from build123d import *

# Parameters (mm, degrees)
SKETCH1_R                 = 5.6
BOSS_EXTRUDE1_DEPTH       = 3
CUT_EXTRUDE1_START        = -3
CUT_EXTRUDE1_DEPTH        = 3
CIRPATTERN1_COUNT         = 12
CIRPATTERN1_START         = -3
CIRPATTERN1_COPY_1_DEPTH  = 3
CIRPATTERN1_COPY_2_DEPTH  = 3
CIRPATTERN1_COPY_3_DEPTH  = 3
CIRPATTERN1_COPY_4_DEPTH  = 3
CIRPATTERN1_COPY_5_DEPTH  = 3
CIRPATTERN1_COPY_6_DEPTH  = 3
CIRPATTERN1_COPY_7_DEPTH  = 3
CIRPATTERN1_COPY_8_DEPTH  = 3
CIRPATTERN1_COPY_9_DEPTH  = 3
CIRPATTERN1_COPY_10_DEPTH = 3
CIRPATTERN1_COPY_11_DEPTH = 3


with BuildPart() as part:
    # Sketch1 → Boss-Extrude1 (new body)
    with BuildSketch(Plane(origin=(0, 0, 0), x_dir=(1, 0, 0), z_dir=(0, 1, 0))):
        with Locations(Location((0, 0, 0), (0, 0, 270))):
            Circle(SKETCH1_R)
    extrude(amount=BOSS_EXTRUDE1_DEPTH)

    # Sketch2 → Cut-Extrude1 (cut)
    with BuildSketch(Plane(origin=(0, 3, 0), x_dir=(1, 0, 0), z_dir=(0, 1, 0)).offset(CUT_EXTRUDE1_START)):
        with BuildLine():
            Line((0.510357412, 3.876549408), (0.730946676, 5.552091224))
            ThreePointArc((0.730946676, 5.552091224), (0.075009446, 5.599497619), (-0.581962275, 5.569678618))
            ThreePointArc((-0.581962275, 5.569678618), (-0.013232679, 4.835071359), (0.066186197, 3.909439779))
            ThreePointArc((0.066186197, 3.909439779), (0.288740502, 3.899324162), (0.510357412, 3.876549408))
        make_face()
    cut_extrude1 = extrude(amount=CUT_EXTRUDE1_DEPTH, mode=Mode.SUBTRACT)

    # Mirror1: Cut-Extrude1 across plane
    add(cut_extrude1.mirror(Plane(origin=(0, 0, 0), x_dir=(-0.13052619222004483, 0, 0.9914448613738113), z_dir=(-0.9914448613738114, 0, -0.13052619222004483))), mode=Mode.SUBTRACT)

    # CirPattern1: Cut-Extrude1 ×12 about axis
    cirpattern1_axis = Axis((0, 0, 0), (0, 1, 0))
    for i in range(1, CIRPATTERN1_COUNT):
        add(cut_extrude1.rotate(cirpattern1_axis, i * 360 / CIRPATTERN1_COUNT), mode=Mode.SUBTRACT)

    # CirPattern1 copy 1 sketch → CirPattern1 copy 1 (cut)
    with BuildSketch(Plane(origin=(0, 3, 0), x_dir=(-0.9659258262890651, 0, 0.25881904510253406), z_dir=(0, 1, 0)).offset(CIRPATTERN1_START)):
        with BuildLine():
            Line((0.510357412, -3.876549408), (0.730946676, -5.552091224))
            ThreePointArc((0.730946676, -5.552091224), (0.075009446, -5.599497619), (-0.581962275, -5.569678618))
            ThreePointArc((-0.581962275, -5.569678618), (-0.013232679, -4.835071359), (0.066186197, -3.909439779))
            ThreePointArc((0.066186197, -3.909439779), (0.288740502, -3.899324162), (0.510357412, -3.876549408))
        make_face()
    extrude(amount=CIRPATTERN1_COPY_1_DEPTH, mode=Mode.SUBTRACT)

    # CirPattern1 copy 2 sketch → CirPattern1 copy 2 (cut)
    with BuildSketch(Plane(origin=(0, 3, 0), x_dir=(-0.7071067811865381, 0, 0.7071067811865575), z_dir=(0, 1, 0)).offset(CIRPATTERN1_START)):
        with BuildLine():
            Line((0.510357412, -3.876549408), (0.730946676, -5.552091224))
            ThreePointArc((0.730946676, -5.552091224), (0.075009446, -5.599497619), (-0.581962275, -5.569678618))
            ThreePointArc((-0.581962275, -5.569678618), (-0.013232679, -4.835071359), (0.066186197, -3.909439779))
            ThreePointArc((0.066186197, -3.909439779), (0.288740502, -3.899324162), (0.510357412, -3.876549408))
        make_face()
    extrude(amount=CIRPATTERN1_COPY_2_DEPTH, mode=Mode.SUBTRACT)

    # CirPattern1 copy 3 sketch → CirPattern1 copy 3 (cut)
    with BuildSketch(Plane(origin=(0, 3, 0), x_dir=(-0.25881904510250764, 0, 0.9659258262890722), z_dir=(0, 1, 0)).offset(CIRPATTERN1_START)):
        with BuildLine():
            Line((0.510357412, -3.876549408), (0.730946676, -5.552091224))
            ThreePointArc((0.730946676, -5.552091224), (0.075009446, -5.599497619), (-0.581962275, -5.569678618))
            ThreePointArc((-0.581962275, -5.569678618), (-0.013232679, -4.835071359), (0.066186197, -3.909439779))
            ThreePointArc((0.066186197, -3.909439779), (0.288740502, -3.899324162), (0.510357412, -3.876549408))
        make_face()
    extrude(amount=CIRPATTERN1_COPY_3_DEPTH, mode=Mode.SUBTRACT)

    # CirPattern1 copy 4 sketch → CirPattern1 copy 4 (cut)
    with BuildSketch(Plane(origin=(0, 3, 0), x_dir=(0.2588190451025339, 0, 0.9659258262890651), z_dir=(0, 1, 0)).offset(CIRPATTERN1_START)):
        with BuildLine():
            Line((0.510357412, -3.876549408), (0.730946676, -5.552091224))
            ThreePointArc((0.730946676, -5.552091224), (0.075009446, -5.599497619), (-0.581962275, -5.569678618))
            ThreePointArc((-0.581962275, -5.569678618), (-0.013232679, -4.835071359), (0.066186197, -3.909439779))
            ThreePointArc((0.066186197, -3.909439779), (0.288740502, -3.899324162), (0.510357412, -3.876549408))
        make_face()
    extrude(amount=CIRPATTERN1_COPY_4_DEPTH, mode=Mode.SUBTRACT)

    # CirPattern1 copy 5 sketch → CirPattern1 copy 5 (cut)
    with BuildSketch(Plane(origin=(0, 3, 0), x_dir=(0.7071067811865577, 0, 0.707106781186538), z_dir=(0, 1, 0)).offset(CIRPATTERN1_START)):
        with BuildLine():
            Line((0.510357412, -3.876549408), (0.730946676, -5.552091224))
            ThreePointArc((0.730946676, -5.552091224), (0.075009446, -5.599497619), (-0.581962275, -5.569678618))
            ThreePointArc((-0.581962275, -5.569678618), (-0.013232679, -4.835071359), (0.066186197, -3.909439779))
            ThreePointArc((0.066186197, -3.909439779), (0.288740502, -3.899324162), (0.510357412, -3.876549408))
        make_face()
    extrude(amount=CIRPATTERN1_COPY_5_DEPTH, mode=Mode.SUBTRACT)

    # CirPattern1 copy 6 sketch → CirPattern1 copy 6 (cut)
    with BuildSketch(Plane(origin=(0, 3, 0), x_dir=(0.9659258262890722, 0, 0.2588190451025077), z_dir=(0, 1, 0)).offset(CIRPATTERN1_START)):
        with BuildLine():
            Line((0.510357412, -3.876549408), (0.730946676, -5.552091224))
            ThreePointArc((0.730946676, -5.552091224), (0.075009446, -5.599497619), (-0.581962275, -5.569678618))
            ThreePointArc((-0.581962275, -5.569678618), (-0.013232679, -4.835071359), (0.066186197, -3.909439779))
            ThreePointArc((0.066186197, -3.909439779), (0.288740502, -3.899324162), (0.510357412, -3.876549408))
        make_face()
    extrude(amount=CIRPATTERN1_COPY_6_DEPTH, mode=Mode.SUBTRACT)

    # CirPattern1 copy 7 sketch → CirPattern1 copy 7 (cut)
    with BuildSketch(Plane(origin=(0, 3, 0), x_dir=(0.9659258262890651, 0, -0.2588190451025343), z_dir=(0, 1, 0)).offset(CIRPATTERN1_START)):
        with BuildLine():
            Line((0.510357412, -3.876549408), (0.730946676, -5.552091224))
            ThreePointArc((0.730946676, -5.552091224), (0.075009446, -5.599497619), (-0.581962275, -5.569678618))
            ThreePointArc((-0.581962275, -5.569678618), (-0.013232679, -4.835071359), (0.066186197, -3.909439779))
            ThreePointArc((0.066186197, -3.909439779), (0.288740502, -3.899324162), (0.510357412, -3.876549408))
        make_face()
    extrude(amount=CIRPATTERN1_COPY_7_DEPTH, mode=Mode.SUBTRACT)

    # CirPattern1 copy 8 sketch → CirPattern1 copy 8 (cut)
    with BuildSketch(Plane(origin=(0, 3, 0), x_dir=(0.7071067811865385, 0, -0.7071067811865571), z_dir=(0, 1, 0)).offset(CIRPATTERN1_START)):
        with BuildLine():
            Line((0.510357412, -3.876549408), (0.730946676, -5.552091224))
            ThreePointArc((0.730946676, -5.552091224), (0.075009446, -5.599497619), (-0.581962275, -5.569678618))
            ThreePointArc((-0.581962275, -5.569678618), (-0.013232679, -4.835071359), (0.066186197, -3.909439779))
            ThreePointArc((0.066186197, -3.909439779), (0.288740502, -3.899324162), (0.510357412, -3.876549408))
        make_face()
    extrude(amount=CIRPATTERN1_COPY_8_DEPTH, mode=Mode.SUBTRACT)

    # CirPattern1 copy 9 sketch → CirPattern1 copy 9 (cut)
    with BuildSketch(Plane(origin=(0, 3, 0), x_dir=(0.25881904510250775, 0, -0.9659258262890722), z_dir=(0, 1, 0)).offset(CIRPATTERN1_START)):
        with BuildLine():
            Line((0.510357412, -3.876549408), (0.730946676, -5.552091224))
            ThreePointArc((0.730946676, -5.552091224), (0.075009446, -5.599497619), (-0.581962275, -5.569678618))
            ThreePointArc((-0.581962275, -5.569678618), (-0.013232679, -4.835071359), (0.066186197, -3.909439779))
            ThreePointArc((0.066186197, -3.909439779), (0.288740502, -3.899324162), (0.510357412, -3.876549408))
        make_face()
    extrude(amount=CIRPATTERN1_COPY_9_DEPTH, mode=Mode.SUBTRACT)

    # CirPattern1 copy 10 sketch → CirPattern1 copy 10 (cut)
    with BuildSketch(Plane(origin=(0, 3, 0), x_dir=(-0.2588190451025343, 0, -0.9659258262890651), z_dir=(0, 1, 0)).offset(CIRPATTERN1_START)):
        with BuildLine():
            Line((0.510357412, -3.876549408), (0.730946676, -5.552091224))
            ThreePointArc((0.730946676, -5.552091224), (0.075009446, -5.599497619), (-0.581962275, -5.569678618))
            ThreePointArc((-0.581962275, -5.569678618), (-0.013232679, -4.835071359), (0.066186197, -3.909439779))
            ThreePointArc((0.066186197, -3.909439779), (0.288740502, -3.899324162), (0.510357412, -3.876549408))
        make_face()
    extrude(amount=CIRPATTERN1_COPY_10_DEPTH, mode=Mode.SUBTRACT)

    # CirPattern1 copy 11 sketch → CirPattern1 copy 11 (cut)
    with BuildSketch(Plane(origin=(0, 3, 0), x_dir=(-0.7071067811865571, 0, -0.7071067811865385), z_dir=(0, 1, 0)).offset(CIRPATTERN1_START)):
        with BuildLine():
            Line((0.510357412, -3.876549408), (0.730946676, -5.552091224))
            ThreePointArc((0.730946676, -5.552091224), (0.075009446, -5.599497619), (-0.581962275, -5.569678618))
            ThreePointArc((-0.581962275, -5.569678618), (-0.013232679, -4.835071359), (0.066186197, -3.909439779))
            ThreePointArc((0.066186197, -3.909439779), (0.288740502, -3.899324162), (0.510357412, -3.876549408))
        make_face()
    extrude(amount=CIRPATTERN1_COPY_11_DEPTH, mode=Mode.SUBTRACT)


solid = part.part
Design review of the part built by this model. Coordinates are the model's own, in mm. A direction names the side the tool comes from. Round coordinates to 2 decimals unless told otherwise and drop trailing zeros. Order: outer loops, then holes, each group sorted by start corner. A loop starts at its lowest first (then second) coordinate and runs counter-clockwise, first axis right, second up. Notation, with made-up numbers: M 11,23 L 27,23 A23 cw 27,47 Z; hole C 23,29 d3. An arc over 180 degrees is marked long. Answer as CSV lines item,"result". Start each with the question number.
1) Wall thickness on line 1 along X through (y, z) = (1.05, 4.25); line 2 along Z through (x, y) = (3, 1.25); line 3 along Z through (x, y) = (-3, 0.4): over which ranges is each line inside the solid? List them lowest first. Write a range as [from, to].
2) The part is to be moulded in two halves that separate along X. For faces 3 (the face through (0, 3, 0)), 4 (the face through (-1.272, 1.479, 4.677)), say which applies: +X half, -X half, draft (parallel to the pull), parting line (faces both ways), or undercut.
3) Add section B-B (x = 1.75). Give the boundary of the cut face in (y, z), then the cut area to 3 significant figures.
4) Tool access review of faces 1 (the face through (4.677, 1.479, 1.272)), 2 (the face through (0, 0, 0)): name each direction out of +Z, -Z, +X, -X, +Y, -Y from which nothing blocks a thin tool from reaching the whole face with its end or side.
5) For pin 1 Ø1 at (x, y) = (-4, 2.5) entering from +Z, flat-tipped, find the tip position at first contact; note if it passes through.
6) Add section A-A (z = -0.25). Give the boundary of the cut face in (x, y).
Resolved:
1,line 1,"[-2.41, -1.04], [-0.1, 1.23], [2.52, 3.54]"
1,line 2,"[-3.14, 2.51], [2.86, 4.48]"
1,line 3,"[-4.48, -2.86], [-2.51, 3.14]"
2,face 3,"draft"
2,face 4,"undercut"
3,outline,"M 0,-5.11 L 3,-5.11 L 3,3.5 L 0,3.5 Z"
3,area,"25.8 mm^2"
4,face 1,"+X, +Y, -Y"
4,face 2,"+Z, -Z, +X, -X, -Y"
5,pin 1,"z = 3.55"
6,outline,"M -3.9,0 L 5.25,0 L 5.25,3 L -3.9,3 Z"
